```python
from build123d import *

# Parameters (mm, degrees)
SKETCH1_R           = 37.5
BOSS_EXTRUDE1_DEPTH = 45
SKETCH5_R           = 36.5
CUT_EXTRUDE2_DEPTH  = 18
CUT_REVOLVE3_ANGLE  = 180
CHAMFER1_SIZE       = 10


with BuildPart() as part:
    # Sketch1 → Boss-Extrude1 (new body)
    with BuildSketch(Plane.XY):
        Circle(SKETCH1_R)
    extrude(amount=BOSS_EXTRUDE1_DEPTH)

    # Sketch5 → Cut-Extrude2 (cut)
    with BuildSketch(Plane.XY.offset(45)):
        Circle(SKETCH5_R)
    extrude(amount=-CUT_EXTRUDE2_DEPTH, mode=Mode.SUBTRACT)

    # Sketch7 → Cut-Revolve3 (revolve, cut)
    with BuildSketch(Plane.XY.offset(27)):
        with BuildLine():
            Line((-36, 0), (36, 0))
            ThreePointArc((36, 0), (0, 36), (-36, 0))
        make_face()
    revolve(axis=Axis((-36, 0, 27), (-1, 0, 0)), revolution_arc=CUT_REVOLVE3_ANGLE, mode=Mode.SUBTRACT)

    # Chamfer1
    chamfer1_edges = [part.edges().sort_by_distance(p)[0] for p in [
        (-37.5, 0, 0),
    ]]
    chamfer(chamfer1_edges, length=CHAMFER1_SIZE)


solid = part.part
```
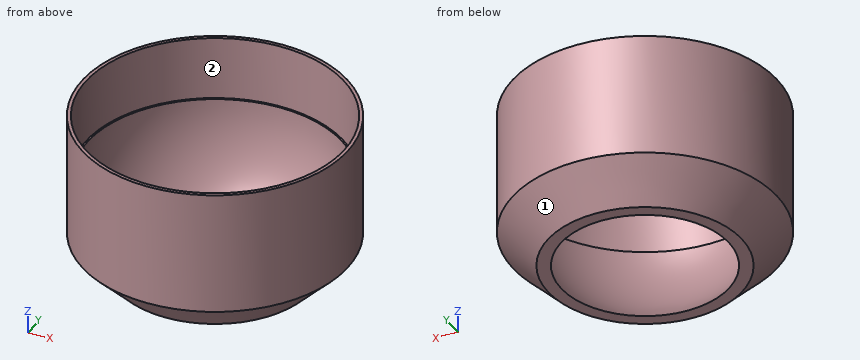
Build history of the part. All positions in model axes, mm. Face numbers are marked on the shaded views. Give positions to 0.01 mm unless a question says otherwise; leave off trailing zeros. Loops run counter-clockwise (first coordinate to the right, second up) from the corner with the lowest first, then second, coordinate; pieces in that order, holes last.
1) Band-saw the part on A-A on y = 0. List the corners of the cut face in (x, z).
Values follow:
outline: (-37.5, 10) - (-27.5, 0) - (-23.81, 0) arc R36 cw to (-36, 27) - (-36.5, 27) - (-36.5, 45) - (-37.5, 45) - close; (23.81, 0) - (27.5, 0) - (37.5, 10) - (37.5, 45) - (36.5, 45) - (36.5, 27) - (36, 27) arc R36 cw to start
2) Band-saw the part on C-C on z = 8. List the corners of the cut face in (x, y).
Values follow:
outline: circle Ø71 at (0, 0); hole circle Ø61.16 at (0, 0)
3) Probe line 1 along Y through (x, z) = (0, 34.75); line 2 along Y through (x, z) = (-12, 23.5); line 3 along Z through (x, y) = (-0.5, -25.5). List the from-to ranges inside material, lowest first.
Values follow:
line 1: y = -37.5 to -36.5, 36.5 to 37.5
line 2: y = -35.53 to -33.76, 33.76 to 35.53
line 3: z = 0 to 1.59
4) Drop flat-ended pins along their axis: P1, Ø8, axis at y = -27, z = 25.5, coming from the +X side; P2, Ø6, axis at y = -1.5, z = 12.5, coming from the +X side; P3, Ø1.5, axis at x = 26.5, z = 13, coming from the -Y side; P4, Ø5, axis at y = -20, z = 26, coming from the +X side. Give the stop position or say it passes through.
Values follow:
P1: stops at x = 29.62
P2: stops at x = 37.5
P3: stops at y = -27.26
P4: stops at x = 33.17
5) Two-plate mould, pull along X, no slides. Class the marked faces 1 and 2: released by +X, released by -X, zero draft, split by the parting line, or undercut.
Values follow:
face 1: split by the parting line
face 2: undercut
